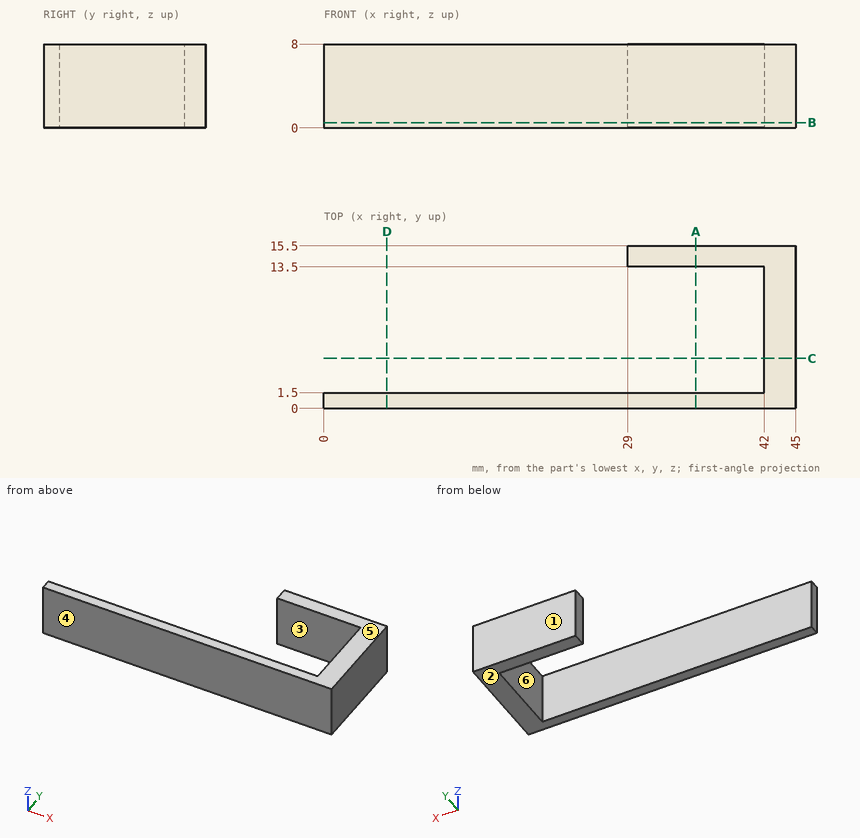
Design review of the part shown in the three views and the two pictorial views. Dimensions are in mm from the part's minimum x, y and z. A direction names the side the tool comes from. Round coordinates to 2 decimals unless told otherwise and drop trailing zeros. Order: outer loops, then holes, each group sorted by start corner. A loop starts at its lowest first (then second) coordinate and runs counter-clockwise, first axis right, second up. Notation, with made-up numbers: M 17,84 L 54,84 A14 cw 54,103 Z; hole C 41.25,-19 d2. An arc over 180 degrees is marked long. Put each result on its own line as item: value.
Q1. Consider section C-C (y = 4.75). State the section outline as (x, z) points, and give its area (3 significant figures).
Reported:
outline: M 42,0 L 45,0 L 45,8 L 42,8 Z
area: 24.0 mm²
Q2. Consider section D-D (x = 6). State the section outline as (y, z) points, and give its area (3 significant figures).
Reported:
outline: M 0,0 L 1.5,0 L 1.5,8 L 0,8 Z
area: 12.0 mm²
Q3. Insertion check: pin 1 Ø4 at (y, z) = (10.5, 1) entering from -X; pin 2 Ø2.5 at (x, z) = (18.5, 3.5) entering from +Y; pin 3 Ø6 at (x, y) = (14, 6) entering from -Z; pin 4 Ø0.6 at (y, z) = (15, 2.5) entering from -X. Each pin has a flat end and moves straight along its axis. Give the tip position at first contact, or say it passes through.
Reported:
pin 1: x = 42
pin 2: y = 1.5
pin 3: through
pin 4: x = 29
Q4. Machinability: for the marked faces 5 and 6, which of the approach directions +Z, -Z, +X, -X, +Y, -Y give a long, thin tool a straight path to every point of the face, cutting with its end or side? Answer none if there is none.
Reported:
face 5: +Z, +X, -X, +Y, -Y
face 6: +Z, -Z, -X
Q5. Draft analysis for pull direction Y (two halves, no side actions). For the marked faces 1, 2, 3 and 4, state which applies: released by +Y, released by -Y, zero draft, split by the parting line, or undercut.
Reported:
face 1: released by +Y
face 2: zero draft
face 3: undercut
face 4: released by -Y
Q6. Consider section A-A (x = 35.5). State the section outline as (y, z) points.
Reported:
outline: M 0,0 L 1.5,0 L 1.5,8 L 0,8 Z; M 13.5,0 L 15.5,0 L 15.5,8 L 13.5,8 Z
Q7. To check wall thickness, follow line 1 (Y direction, x = 30.5, z = 4.5); line 2 (X direction, y = 2, z = 2); line 3 (Y direction, x = 16, z = 1). State the ranges of each line that lie inside material, in increasing order.
Reported:
line 1: 0 to 1.5, 13.5 to 15.5
line 2: 42 to 45
line 3: 0 to 1.5
Q8. Consider section B-B (z = 0.5). State the section outline as (x, y) points.
Reported:
outline: M 0,0 L 45,0 L 45,15.5 L 29,15.5 L 29,13.5 L 42,13.5 L 42,1.5 L 0,1.5 Z
